Input: part model. Units: mm. Frame: model coordinates. A direction names the side the tool comes from. Give positions to 0.01 mm unless a question says otherwise; leave off trailing zeros. Loops run counter-clockwise (first coordinate to the right, second up) from the corner with the lowest first, then second, coordinate; pieces in that order, holes last.
Autodesk Inventor part; units mm, degrees
ref_plane "YZ Plane" through (0, 0, 0) normal (1, 0, 0) x (0, 1, 0)
ref_plane "XZ Plane" through (0, 0, 0) normal (0, 1, 0) x (-1, 0, 0)
ref_plane "XY Plane" through (0, 0, 0) normal (0, 0, 1) x (1, 0, 0)
sketch "Boceto1" plane through (0, 0, 0) normal (0, 1, 0) x (-1, 0, 0)
  line L0 (-10.7233, 10.25) -> (10.7233, 10.25)
  line L1 (10.7233, 10.25) -> (10.7233, -10.25)
  line L2 (10.7233, -10.25) -> (-10.7233, -10.25)
  line L3 (-10.7233, -10.25) -> (-10.7233, 10.25)
  line L4 (-10.7233, 10.25) -> (10.7233, -10.25) construction
  line L5 (10.7233, 10.25) -> (-10.7233, -10.25) construction
  line L6 (-10.7233, 12.25) -> (10.7233, 12.25)
  line L7 (10.7233, 12.25) -> (10.7233, -12.25)
  line L8 (10.7233, -12.25) -> (-10.7233, -12.25)
  line L9 (-10.7233, -12.25) -> (-10.7233, 12.25)
  line L10 (-10.7233, 12.25) -> (10.7233, -12.25) construction
  line L11 (10.7233, 12.25) -> (-10.7233, -12.25) construction
  line L12 (10.7233, 12.25) -> (24.7233, 12.25)
  line L13 (24.7233, 12.25) -> (24.7233, -12.25)
  line L14 (24.7233, -12.25) -> (10.7233, -12.25)
  line L15 (10.7233, -12.25) -> (10.7233, 12.25)
  line L16 (10.7233, 10.25) -> (24.7233, 10.25)
  line L17 (24.7233, 10.25) -> (24.7233, -10.25)
  line L18 (24.7233, -10.25) -> (10.7233, -10.25)
  line L19 (10.7233, -10.25) -> (10.7233, 10.25)
  line L20 (24.7233, 12.25) -> (29.2233, 12.25)
  line L21 (29.2233, 12.25) -> (29.2233, -12.25)
  line L22 (29.2233, -12.25) -> (24.7233, -12.25)
  line L23 (24.7233, -12.25) -> (24.7233, 12.25)
  point P0 (0, 0)
  point P1 (24.7233, 10.25)
  point P2 (-10.7233, -10.25)
  dimension "d0" = 20.5
  dimension "d1" = 2
  dimension "d2" = 14
  dimension "d3" = 18.5
extrude "Extrusión1" add sketch "Boceto1" along normal blind 16 contours L9 L6 L7 L0 | L7 L12 L13 L16 | L2 L7 L8 L9 | L18 L13 L14 L7 | L13 L20 L21 L22
sketch "Boceto2" plane through (-29.2233, 0, -12.25) normal (-1, 0, 0) x (0, 0, 1)
  circle A0 centre (7.5, 3.3) radius 1.15
  circle A1 centre (7.5, 12.8) radius 1.15
  line L0 (0, 0) -> (24.5, 0)
  line L1 (0, 0) -> (0, 16)
  point P0 (12.25, 0)
  dimension "d6" = 2.3
  dimension "d7" = 3.3
  dimension "d8" = 9.5
  dimension "d9" = 7.5
extrude "Extrusión2" cut sketch "Boceto2" against normal through all
sketch "Boceto3" plane through (-24.7233, 0, 10.25) normal (1, 0, 0) x (0, 0, -1)
  circle A0 centre (15, 12.8) radius 1.15
  circle A1 centre (15, 12.8) radius 2.15
  circle A2 centre (15, 3.3) radius 1.15
  circle A3 centre (15, 3.3) radius 2.15
  line L0 (17.4826, 12.8) -> (16.2413, 10.65)
  line L1 (16.2413, 10.65) -> (13.7587, 10.65)
  line L2 (13.7587, 10.65) -> (12.5174, 12.8)
  line L3 (12.5174, 12.8) -> (13.7587, 14.95)
  line L4 (13.7587, 14.95) -> (16.2413, 14.95)
  line L5 (16.2413, 14.95) -> (17.4826, 12.8)
  line L6 (17.4826, 3.3) -> (16.2413, 1.15)
  line L7 (16.2413, 1.15) -> (13.7587, 1.15)
  line L8 (13.7587, 1.15) -> (12.5174, 3.3)
  line L9 (12.5174, 3.3) -> (13.7587, 5.45)
  line L10 (13.7587, 5.45) -> (16.2413, 5.45)
  line L11 (16.2413, 5.45) -> (17.4826, 3.3)
  point P0 (10.25, 0)
  dimension "d12" = 4.3
extrude "Extrusión3" cut sketch "Boceto3" against normal blind 2.5 contours A0 | A1 | A1 L5 L0 | A1 L4 L5 | L0 L1 A1 | A1 L3 L4 | L1 L2 A1 | A1 L2 L3 | A2 | A3 | A3 L11 L6 | A3 L10 L11 | L6 L7 A3 | A3 L9 L10 | L7 L8 A3 | A3 L8 L9
sketch "Boceto4" plane through (-29.2233, 0, 12.25) normal (0, 0, 1) x (1, 0, 0)
  circle A0 centre (29.9467, 8) radius 2.7
  line L0 (39.9467, 0) -> (39.9467, 16)
  line L1 (0, 0) -> (39.9467, 0)
  point P0 (29.2233, 0)
  dimension "d15" = 10
  dimension "d16" = 8
  dimension "d17" = 5.4
extrude "Extrusión4" cut sketch "Boceto4" against normal through all
fillet "Empalme1" radius 2 6 edges at (10.7233, 0, 11.25) (10.7233, 16, 11.25) (10.7233, 16, -11.25) (10.7233, 0, -11.25) (-29.2233, 8, 12.25) (-29.2233, 8, -12.25)
properties part number "gfdsgfd"
(1) Mould query, pull axis Y, two halves, no side actions, for faces 4 (the flat face through (-25.956, 13.89, -6.603)), 5 (the flat face through (-9, 8, -12.25)), 6 (the flat face through (-26, 16, -1)), 7 (the flat face through (-25.96, 11.74, -6.62)). Classes: +Y half, -Y half, draft (parallel to the pull), parting line (faces both ways), or undercut.
Values follow:
face 4: undercut
face 5: draft
face 6: +Y half
face 7: undercut
(2) Cut plane D-D (z = -7.75). Return the cut outline in (x, y), and give its area (3 significant figures).
Values follow:
outline: (-29.22, 0) - (-24.72, 0) - (-24.72, 16) - (-29.22, 16) - close
area: 72.0 mm2
(3) Cut plane C-C (z = -4.75). Return the cut outline in (x, y), and give its area (3 significant figures).
Values follow:
outline: (-29.22, 0) - (-24.72, 0) - (-24.72, 1.15) - (-27.22, 1.15) - (-27.22, 2.15) - (-29.22, 2.15) - close; (-29.22, 4.45) - (-27.22, 4.45) - (-27.22, 5.45) - (-24.72, 5.45) - (-24.72, 10.65) - (-27.22, 10.65) - (-27.22, 11.65) - (-29.22, 11.65) - close; (-29.22, 13.95) - (-27.22, 13.95) - (-27.22, 14.95) - (-24.72, 14.95) - (-24.72, 16) - (-29.22, 16) - close
area: 41.3 mm2
(4) Pin query (flat end, axial travel): pin 1 Ø8 at (y, z) = (11, 0) entering from +X; pin 2 Ø2 at (y, z) = (2.5, -4.5) entering from +X. Return the tip coordinate at first contact, or that it passes through.
Values follow:
pin 1: stops at x = -24.72
pin 2: stops at x = -27.22
(5) Cut plane A-A (x = -19). Return the cut outline in (y, z), and give its area (3 significant figures).
Values follow:
outline: (0, -12.25) - (16, -12.25) - (16, -10.25) - (0, -10.25) - close; (0, 10.25) - (16, 10.25) - (16, 12.25) - (0, 12.25) - close
area: 64.0 mm2
(6) Reachability of faces 1 (the flat face through (-24.723, 8, 0)), 2 (the cylindrical face through (10.12, 0.57, 11.26)), 3 (the flat face through (-26, 10.65, -5)) from +Z, -Z, +X, -X, +Y, -Y: full face, straight path, thin tool, end or side. Return the list, or none.
Values follow:
face 1: +X, +Y, -Y
face 2: +Z, -Z, +X, -Y
face 3: +X
(7) Ray query, probe 1 along Y at (x, z) = (-27, -4); probe 2 along Y at (x, z) = (-28.7, -4.75); probe 3 along Z at (x, y) = (-3, 12). Return the intervals inside material, ascending.
Values follow:
probe 1: y = 0 to 1.15, 5.45 to 10.65, 14.95 to 16
probe 2: y = 0 to 2.15, 4.45 to 11.65, 13.95 to 16
probe 3: z = -12.25 to -10.25, 10.25 to 12.25
(8) Cut plane B-B (y = 8). Return the cut outline in (x, z), and give its area (3 significant figures).
Values follow:
outline: (-29.22, -10.25) arc R2 ccw to (-27.22, -12.25) - (-1.98, -12.25) - (-1.98, -10.25) - (-24.72, -10.25) - (-24.72, 10.25) - (-1.98, 10.25) - (-1.98, 12.25) - (-27.22, 12.25) arc R2 ccw to (-29.22, 10.25) - close; (3.42, -12.25) - (10.72, -12.25) - (10.72, -10.25) - (3.42, -10.25) - close; (3.42, 10.25) - (10.72, 10.25) - (10.72, 12.25) - (3.42, 12.25) - close
area: 229 mm2
